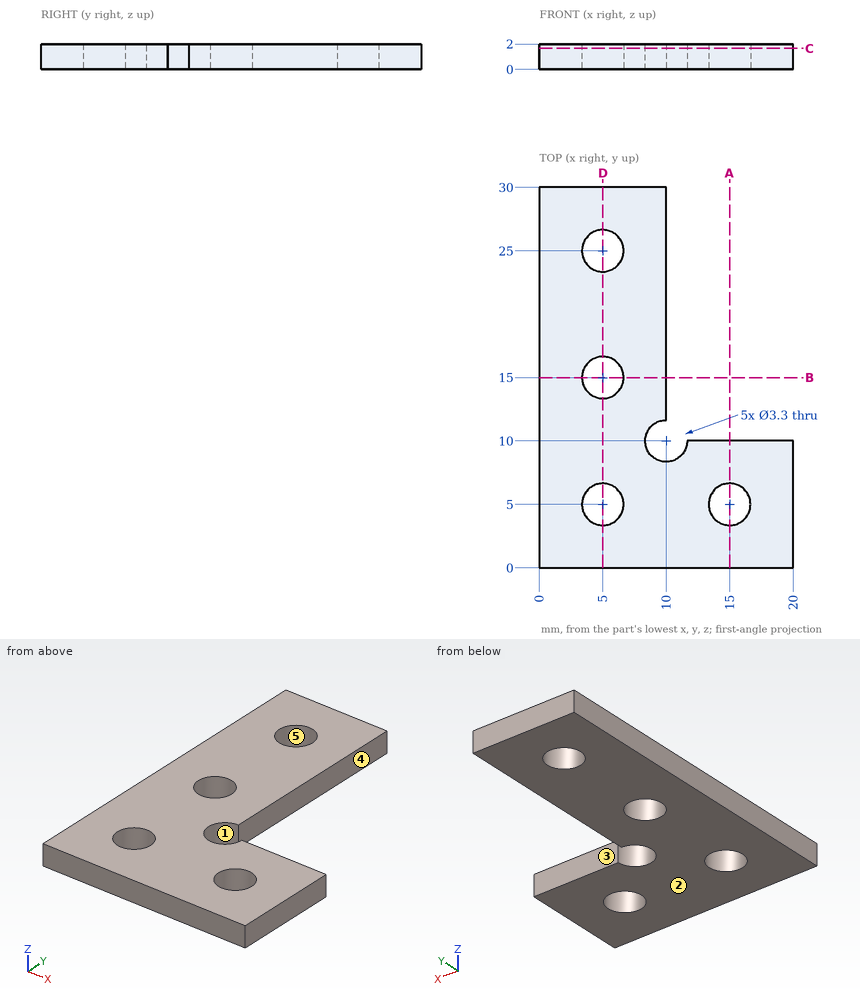
Design review of the part shown in the three views and the two pictorial views. Dimensions are in mm from the part's minimum x, y and z. A direction names the side the tool comes from. Round coordinates to 2 decimals unless told otherwise and drop trailing zeros. Loops run counter-clockwise (first coordinate to the right, second up) from the corner with the lowest first, then second, coordinate; pieces in that order, holes last. Notation, with made-up numbers: (10, 75.25) -> (22, 75.25) arc R19 cw to (22, 85.25) -> close; hole circle Ø7 at (-25.5, 58). An arc over 180 degrees is marked (long way). Use one line per item in the form item = value. Start each with the question number.
Q1. We need section C-C on z = 1.65. Give the boundary of the cut face in (x, y), then the cut area to 3 significant figures.
Q2. We need section D-D on x = 5. Give the boundary of the cut face in (y, z).
Q3. We need section A-A on x = 15. Give the boundary of the cut face in (y, z).
Q4. Wall thickness on line 1 along Y through (x, z) = (5, 1.25); line 2 along Y through (x, z) = (4.25, 0.65); line 3 along X through (y, z) = (25.25, 0.45): over which ranges is each line inside the solid? List them lowest first. Write a range as [from, to].
Q5. Draft analysis for pull direction Y (two halves, no side actions). For the marked faces 1, 2 and 3, state which applies: +Y half, -Y half, draft (parallel to the pull), parting line (faces both ways), or undercut.
Q6. Machinability: for the marked faces 4 and 5, which of the approach directions +Z, -Z, +X, -X, +Y, -Y give a long, thin tool a straight path to every point of the face, cutting with its end or side? Answer none if there is none.
Q7. For pin 1 Ø2.5 at (x, y) = (5, 25) entering from +Z; pin 2 Ø0.6 at (x, z) = (17.5, 1.5) entering from +Y; pin 3 Ø1 at (y, z) = (19.5, 1) entering from +X, all flat-tipped, find the tip position at first contact; note any pin that passes through.
Calculated:
q1.outline = (0, 0) -> (20, 0) -> (20, 10) -> (11.65, 10) arc R1.65 cw (long way) to (10, 11.65) -> (10, 30) -> (0, 30) -> close; hole circle Ø3.3 at (5, 5); hole circle Ø3.3 at (5, 15); hole circle Ø3.3 at (5, 25); hole circle Ø3.3 at (15, 5)
q1.area = 359 mm²
q2.outline = (0, 0) -> (3.35, 0) -> (3.35, 2) -> (0, 2) -> close; (6.65, 0) -> (13.35, 0) -> (13.35, 2) -> (6.65, 2) -> close; (16.65, 0) -> (23.35, 0) -> (23.35, 2) -> (16.65, 2) -> close; (26.65, 0) -> (30, 0) -> (30, 2) -> (26.65, 2) -> close
q3.outline = (0, 0) -> (3.35, 0) -> (3.35, 2) -> (0, 2) -> close; (6.65, 0) -> (10, 0) -> (10, 2) -> (6.65, 2) -> close
q4.line_1 = [0, 3.35], [6.65, 13.35], [16.65, 23.35], [26.65, 30]
q4.line_2 = [0, 3.53], [6.47, 13.53], [16.47, 23.53], [26.47, 30]
q4.line_3 = [0, 3.37], [6.63, 10]
q5.face_1 = undercut
q5.face_2 = draft
q5.face_3 = +Y half
q6.face_4 = +Z, -Z, +X, +Y
q6.face_5 = +Z, -Z
q7.pin_1 = through
q7.pin_2 = 10
q7.pin_3 = 10
